Job drawing, mm, ordinate dimensions from the low corner. One solid piece. A direction names the side the tool comes from. Round coordinates to 2 decimals unless told otherwise and drop trailing zeros. Order: outer loops, then holes, each group sorted by start corner. A loop starts at its lowest first (then second) coordinate and runs counter-clockwise, first axis right, second up. Notation, with made-up numbers: (7, 66.5) -> (42, 66.5) arc R26 cw to (42, 97.5) -> close; hole circle Ø4 at (17.25, 64). An arc over 180 degrees is marked (long way). Return JSON: item names as keys, results as strings. Group by question number.
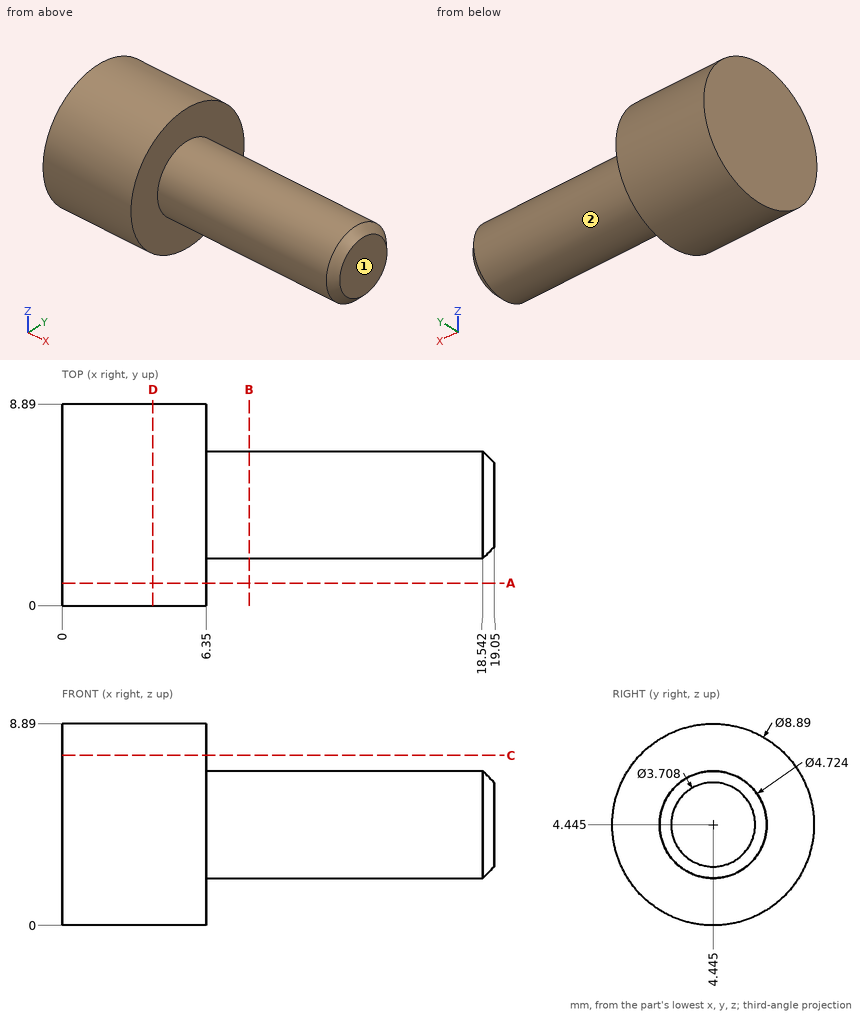
(1) Pin check, flat tips, straight feed: P1, Ø1.5, axis at x = 12, z = 2, coming from the -Y side; P2, Ø3, axis at x = 14.5, y = 6.5, coming from the +Z side; P3, Ø3, axis at x = 10.5, z = 7.5, coming from the +Y side. Stop position of each tip, or through.
(2) Probe L1, parallel to X at y = 8, z = 3.5; L2, parallel to Z at x = 6.25, y = 4.25 (1 decimal); L3, parallel to Y at x = 1, z = 6.25. List the from-to ranges inside material, lowest first. Write a range as [from, to].
(3) Saw through at A-A, the plane y = 1. List the corners of the cut face in (x, z), and give its area (3 significant figures).
(4) Tool access for the marked faces 1 and 2: list every direction of +Z, -Z, +X, -X, +Y, -Y with a clear straight run to the whole face (end or side of a thin tool).
(5) Saw through at B-B, the plane x = 8.25. List the corners of the cut face in (y, z) (1 decimal), and give its area (3 significant figures).
(6) Saw through at C-C, the plane z = 7.5. List the corners of the cut face in (x, y), and give its area (3 significant figures).
(7) Saw through at D-D, the plane x = 4. List the corners of the cut face in (y, z) (1 decimal).
Results are:
{
 "1": {"P1": "stops at y = 2.8", "P2": "stops at z = 6.74", "P3": "stops at y = 6.22"},
 "2": {"L1": "x = [0, 6.35]", "L2": "z = [0, 8.9]", "L3": "y = [0.38, 8.51]"},
 "3": {"outline": "(0, 1.64) -> (6.35, 1.64) -> (6.35, 7.25) -> (0, 7.25) -> close", "area": "35.7 mm^2"},
 "4": {"face 1": "+Z, -Z, +X, +Y, -Y", "face 2": "+X"},
 "5": {"outline": "circle Ø4.7 at (4.4, 4.4)", "area": "17.5 mm^2"},
 "6": {"outline": "(0, 1.22) -> (6.35, 1.22) -> (6.35, 7.67) -> (0, 7.67) -> close", "area": "41.0 mm^2"},
 "7": {"outline": "circle Ø8.9 at (4.4, 4.4)"}
}
